from build123d import *

# Parameters (mm, degrees)
BOSS_EXTRUDE1_DEPTH = 1.5
SKETCH1_3_R         = 2
BOSS_EXTRUDE2_DEPTH = 4


with BuildPart() as part:
    # Sketch1 → Boss-Extrude1 (new body)
    with BuildSketch(Plane.XY):
        with BuildLine():
            Line((-0.965077795, 3.3973761), (-14.211482552, 1.988787352))
            ThreePointArc((-14.211482552, 1.988787352), (-16, 0), (-14.211482552, -1.988787352))
            Line((-14.211482552, -1.988787352), (-0.965077795, -3.3973761))
            ThreePointArc((-0.965077795, -3.3973761), (0.000431807, -3.453017023), (0.966800983, -3.415131426))
            Line((0.966800983, -3.415131426), (17.174893203, -1.992338417))
            ThreePointArc((17.174893203, -1.992338417), (19, 0), (17.174893203, 1.992338417))
            Line((17.174893203, 1.992338417), (0.966800983, 3.415131426))
            ThreePointArc((0.966800983, 3.415131426), (0.000431807, 3.453017023), (-0.965077795, 3.3973761))
        make_face()
    extrude(amount=BOSS_EXTRUDE1_DEPTH)

    # Sketch1<3> → Boss-Extrude2 (add)
    with BuildSketch(Plane.XY):
        with BuildLine():
            ThreePointArc((0.65921534, 3.437358744), (-0.048694481, 3.452444827), (-0.755897232, 3.417399505))
            ThreePointArc((-0.755897232, 3.417399505), (-3.5, 0), (-0.755897232, -3.417399505))
            ThreePointArc((-0.755897232, -3.417399505), (-0.048694481, -3.452444827), (0.65921534, -3.437358744))
            ThreePointArc((0.65921534, -3.437358744), (2.697893038, -2.229657632), (3.5, 0))
            ThreePointArc((3.5, 0), (2.697893038, 2.229657632), (0.65921534, 3.437358744))
        make_face()
        Circle(SKETCH1_3_R, mode=Mode.SUBTRACT)
    extrude(amount=BOSS_EXTRUDE2_DEPTH)


solid = part.part
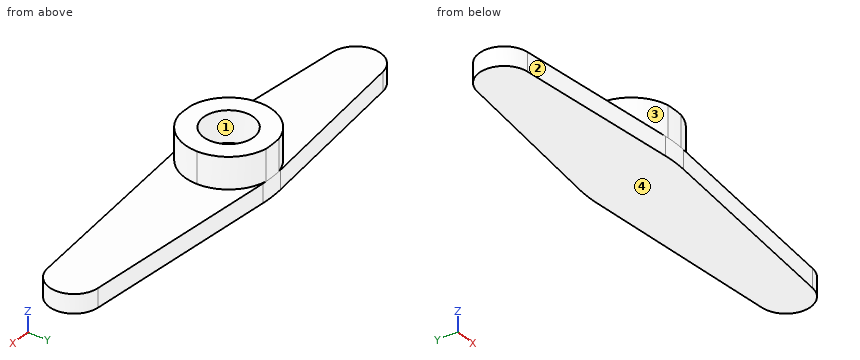
Part model, mm, in its own coordinate system. Face numbers are marked on the shaded views. Give positions to 0.01 mm unless a question says otherwise; leave off trailing zeros. Loops run counter-clockwise (first coordinate to the right, second up) from the corner with the lowest first, then second, coordinate; pieces in that order, holes last. Notation, with made-up numbers: M 72,76.5 L 126,76.5 A31 cw 126,102.5 Z; hole C 62.25,61.5 d3. An arc over 180 degrees is marked long. Put each result on its own line as item: value. Start each with the question number.
1) Saw through at A-A (z = 0.35). List the corners of the cut face in (x, y), then the cut area to 3 significant figures.
2) Pull direction Y, two halves, no side cores. Call the marked faces 1, 2, 3 and 4: +Y half, -Y half, draft (parallel to the pull), parting line (faces both ways), or undercut.
3) Saw through at C-C (x = -1.5). List the corners of the cut face in (y, z).
4) Saw through at D-D (y = 0.5). List the corners of the cut face in (x, z), then the cut area to 3 significant figures.
5) Flat gauge pins, fed straight in: pin 1 (1 mm diameter, centred on x = 14.5, y = -2, fed in from +Z); pin 2 (3 mm diameter, centred on x = 1, y = 0.5, fed in from +Z). Where does each tip first touch, or does it go through?
6) Probe probe 1 along X at (y, z) = (0, 3.1); probe 2 along Y at (x, z) = (0, 2.65); probe 3 along Z at (x, y) = (-3.5, 0.5). List the from-to ranges inside material, lowest first.
7) Saw through at B-B (z = 3.15). List the corners of the cut face in (x, y), then the cut area to 3 significant figures.
Numbers:
1. outline: M -14.21,-1.99 L -0.97,-3.4 A10 ccw 0.97,-3.42 L 17.17,-1.99 A2 ccw 17.17,1.99 L 0.97,3.42 A10 ccw -0.97,3.4 L -14.21,1.99 A2 ccw Z
1. area: 183 mm^2
2. face 1: undercut
2. face 2: -Y half
2. face 3: parting line
2. face 4: draft
3. outline: M -3.34,0 L 3.34,0 L 3.34,1.5 L 3.16,1.5 L 3.16,4 L 1.32,4 L 1.32,1.5 L -1.32,1.5 L -1.32,4 L -3.16,4 L -3.16,1.5 L -3.34,1.5 Z
4. outline: M -15.94,0 L 18.94,0 L 18.94,1.5 L 3.46,1.5 L 3.46,4 L 1.94,4 L 1.94,1.5 L -1.94,1.5 L -1.94,4 L -3.46,4 L -3.46,1.5 L -15.94,1.5 Z
4. area: 59.9 mm^2
5. pin 1: z = 1.5
5. pin 2: z = 4
6. probe 1: -3.5 to -2, 2 to 3.5
6. probe 2: -3.45 to -2, 2 to 3.45
6. probe 3: 0 to 1.5
7. outline: M -0.76,-3.42 A10 ccw 0.66,-3.44 A3.5 ccw 0.66,3.44 A10 ccw -0.76,3.42 A3.5 ccw Z; hole C 0,0 d4
7. area: 25.8 mm^2
